The model under review builds one solid part; all positions refer to its coordinate system, in mm. Face numbers are marked on the shaded views. A direction names the side the tool comes from. Round coordinates to 2 decimals unless told otherwise and drop trailing zeros. Loops run counter-clockwise (first coordinate to the right, second up) from the corner with the lowest first, then second, coordinate; pieces in that order, holes last. Notation, with made-up numbers: M -40,-28 L -13,-28 A22 cw -13,-17 Z; hole C 41.5,51.25 d11. An arc over 180 degrees is marked long. Use a Markdown table: item, result. Add a question column.
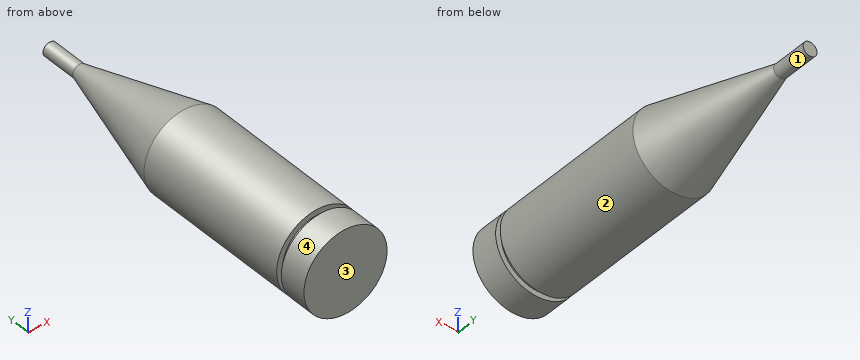
```python
from build123d import *


with BuildPart() as part:
    # Croquis1 → Revolución1 (revolve)
    with BuildSketch(Plane.XY, mode=Mode.PRIVATE) as revoluci_n1_sk:
        Polygon((0, 130), (0, 0), (15, 0), (15, 10), (13, 10), (13, 12), (15, 12), (15, 70.349364905), (2.5, 117), (2.5, 130), align=None)
    revolve(revoluci_n1_sk.sketch.rotate(Axis((0, 130, 0), (0, -1, 0)), 180), axis=Axis((0, 130, 0), (0, -1, 0)))


solid = part.part
```
(1) Insertion check: pin 1 Ø2 at (x, y) = (-11, 37) entering from -Z; pin 2 Ø5 at (x, y) = (-7, 30) entering from -Z; pin 3 Ø1 at (x, y) = (11.5, 53) entering from -Z. Each pin has a flat end and moves straight along its axis. Give the tip position at first contact, or say it passes through.
(2) Consider section B-B, the plane x = 0. Give the boundary of the cut face in (y, z).
(3) Draft analysis for pull direction X (two halves, no side actions). For the marked faces 3 and 4, state which applies: released by +X, released by -X, zero draft, split by the parting line, or undercut.
(4) To check wall thickness, follow probe 1 along X at (y, z) = (59, 0.5); probe 2 along X at (y, z) = (81, 9.25); probe 3 along Z at (x, y) = (-6.5, 19.5). State the ranges of each line that lie inside material, in increasing order.
(5) Consider section A-A, the plane z = 0. Give the boundary of the cut face in (x, y), then the cut area to 3 significant figures.
(6) Consider section C-C, the plane y = 20. Give the boundary of the cut face in (x, z), then the cut area to 3 significant figures.
(7) Consider section D-D, the plane y = 73.5. Give the boundary of the cut face in (x, z).
(8) For the marked faces 1 and 2, list the 3-axis set-ups (+Z, -Z, +X, -X, +Y, -Y) from which the entire face can be reached by the end or side of a thin tool; tool diameter is ignored.
Found:
| question | item | result |
|---|---|---|
| 1 | pin 1 | stops at z = -11.18 |
| 1 | pin 2 | stops at z = -14.31 |
| 1 | pin 3 | stops at z = -10.2 |
| 2 | outline | M 0,-15 L 10,-15 L 10,-13 L 12,-13 L 12,-15 L 70.35,-15 L 117,-2.5 L 130,-2.5 L 130,2.5 L 117,2.5 L 70.35,15 L 12,15 L 12,13 L 10,13 L 10,15 L 0,15 Z |
| 3 | face 3 | zero draft |
| 3 | face 4 | split by the parting line |
| 4 | probe 1 | x = -14.99 to 14.99 |
| 4 | probe 2 | x = -7.87 to 7.87 |
| 4 | probe 3 | z = -13.52 to 13.52 |
| 5 | outline | M -15,0 L 15,0 L 15,10 L 13,10 L 13,12 L 15,12 L 15,70.35 L 2.5,117 L 2.5,130 L -2.5,130 L -2.5,117 L -15,70.35 L -15,12 L -13,12 L -13,10 L -15,10 Z |
| 5 | area | 2,980 mm^2 |
| 6 | outline | C 0,0 d30 |
| 6 | area | 707 mm^2 |
| 7 | outline | C 0,0 d28.31 |
| 8 | face 1 | +Y |
| 8 | face 2 | +Y, -Y |
